The figure shows three views and two pictorial views of one solid part (mm, origin at its lowest corner). Answer the questions. Round coordinates to 2 decimals unless told otherwise and drop trailing zeros. Order: outer loops, then holes, each group sorted by start corner. A loop starts at its lowest first (then second) coordinate and runs counter-clockwise, first axis right, second up. Notation, with made-up numbers: (54.25, 37) - (99.25, 37) arc R21 ccw to (99.25, 62) - close; hole circle Ø4 at (84.5, 10). An arc over 180 degrees is marked (long way). One line per question, with ' | ' between items. Start each with the question number.
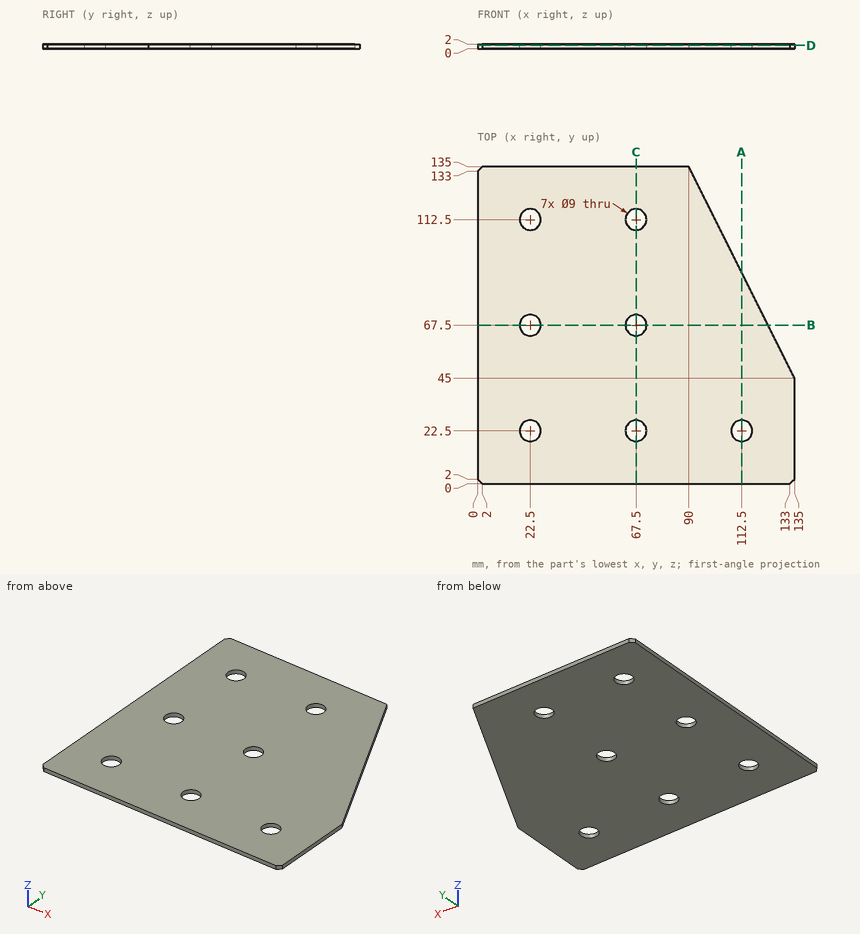
1) Section D-D on z = 1.4 is taken. Give the vertices of the cut face in (x, y).
2) Section C-C on x = 67.5 is taken. Give the vertices of the cut face in (y, z), and give its area (3 significant figures).
3) Straight lines are drawn through the part: line 1 (X direction, y = 22.5, z = 0.7); line 2 (Y direction, x = 112.5, z = 1). For each, find the intervals that lie inside material, in ascending order.
4) Section B-B on y = 67.5 is taken. Give the vertices of the cut face in (x, z).
5) A flat-ended cylindrical pin translates along its axis: pin 1 (8 mm diameter, centred on x = 104, y = 120, fed in from +Z). Find the tip coordinate at first contact, or state that the pin passes through.
6) Section A-A on x = 112.5 is taken. Give the vertices of the cut face in (y, z), and give its area (3 significant figures).
Recorded:
1) outline: (0, 2) - (2, 0) - (133, 0) - (135, 2) - (135, 45) - (90, 135) - (2, 135) - (0, 133) - close; hole circle Ø9 at (22.5, 22.5); hole circle Ø9 at (22.5, 67.5); hole circle Ø9 at (22.5, 112.5); hole circle Ø9 at (67.5, 22.5); hole circle Ø9 at (67.5, 67.5); hole circle Ø9 at (67.5, 112.5); hole circle Ø9 at (112.5, 22.5)
2) outline: (0, 0) - (18, 0) - (18, 2) - (0, 2) - close; (27, 0) - (63, 0) - (63, 2) - (27, 2) - close; (72, 0) - (108, 0) - (108, 2) - (72, 2) - close; (117, 0) - (135, 0) - (135, 2) - (117, 2) - close | area: 216 mm²
3) line 1: x = 0 to 18, 27 to 63, 72 to 108, 117 to 135 | line 2: y = 0 to 18, 27 to 90
4) outline: (0, 0) - (18, 0) - (18, 2) - (0, 2) - close; (27, 0) - (63, 0) - (63, 2) - (27, 2) - close; (72, 0) - (123.75, 0) - (123.75, 2) - (72, 2) - close
5) pin 1: passes through
6) outline: (0, 0) - (18, 0) - (18, 2) - (0, 2) - close; (27, 0) - (90, 0) - (90, 2) - (27, 2) - close | area: 162 mm²
